from build123d import *

# Parameters (mm, degrees)
F0_W     = 25.3558125973
F0_H     = 19.05
F1_DEPTH = 63.5


with BuildPart() as f1:
    # F0 (on Front) → F1 (new body, symmetric)
    with BuildSketch(Plane.XZ):
        with BuildLine():
            add(Edge.make_bspline(
                [(-41.275, 9.525), (-35.7851044723, 45.3244073821), (12.6259092466, 60.7791905255), (51.7188934867, 61.909732843)],
                knots=[0, 0, 0, 0, 106.3505390395, 106.3505390395, 106.3505390395, 106.3505390395], degree=3))
            Line((-41.275, 9.525), (22.225, 9.525))
            Line((22.225, 9.525), (22.225, 27.4096066543))
            ThreePointArc((22.225, 27.4096066543), (30.6034651981, 50.1040358168), (51.7188934867, 61.909732843))
        make_face()
        Polygon((22.225, 9.525), (-41.275, 9.525), (-41.275, -9.525), (41.275, -9.525), (41.275, 9.525), align=None)
        with BuildLine():
            Line((22.225, 27.4096066543), (22.225, 9.525))
            Line((22.225, 9.525), (41.275, 9.525))
            Line((41.275, 9.525), (41.275, 27.4096066543))
            ThreePointArc((41.275, 27.4096066543), (44.7225989891, 37.2876291848), (53.567954849, 42.8752))
            Line((53.567954849, 42.8752), (60.325, 42.8752))
            Line((60.325, 42.8752), (60.325, 61.9252))
            Line((60.325, 61.9252), (52.2881304538, 61.9252))
            add(Edge.make_bspline(
                [(51.7188934867, 61.909732843), (51.9088611725, 61.9152265783), (52.0986088263, 61.9203820671), (52.2881304538, 61.9252)],
                knots=[106.3505390395, 106.3505390395, 106.3505390395, 106.3505390395, 106.8673367765, 106.8673367765, 106.8673367765, 106.8673367765], degree=3))
            ThreePointArc((51.7188934867, 61.909732843), (30.6034651981, 50.1040358168), (22.225, 27.4096066543))
        make_face()
        with BuildLine():
            ThreePointArc((51.8180734259, 61.9252), (51.7684778995, 61.9175020535), (51.7188934867, 61.909732843))
            add(Edge.make_bspline(
                [(51.7188934867, 61.909732843), (51.9088611725, 61.9152265783), (52.0986088263, 61.9203820671), (52.2881304538, 61.9252)],
                knots=[106.3505390395, 106.3505390395, 106.3505390395, 106.3505390395, 106.8673367765, 106.8673367765, 106.8673367765, 106.8673367765], degree=3))
            Line((52.2881304538, 61.9252), (51.8180734259, 61.9252))
        make_face()
        with BuildLine():
            add(Edge.make_bspline(
                [(52.2881304538, 61.9252), (55.0200364706, 61.994649277), (57.7049776323, 61.993959567), (60.325, 61.9252)],
                knots=[106.8673367765, 106.8673367765, 106.8673367765, 106.8673367765, 114.3168446032, 114.3168446032, 114.3168446032, 114.3168446032], degree=3))
            Line((52.2881304538, 61.9252), (60.325, 61.9252))
        make_face()
        with Locations((73.0029062986, 52.4002)):
            Rectangle(F0_W, F0_H)
        Polygon((60.325, 66.675), (60.325, 61.9252), (85.6808125973, 61.9252), (85.6808125973, 42.8752), (60.325, 42.8752), (60.325, 38.1), (111.125, 38.1), (111.125, 66.675), align=None)
    extrude(amount=F1_DEPTH, both=True)


solid = f1.part
Part model, mm, in its own coordinate system. A direction names the side the tool comes from. Round coordinates to 2 decimals unless told otherwise and drop trailing zeros. Write each loop counter-clockwise with the first axis right and the second up, starting at its lowest first coordinate (ties: lowest second). Pieces come first, ordered by that corner, then holes. Notation, with made-up numbers: M 60.25,62 L 97.25,62 A13 cw 97.25,74 Z; hole C 26,9 d9. An arc over 180 degrees is marked long. Return JSON: item names as keys, results as strings. Group by question number.
(1) Which spindle directions (+Z, -Z, +X, -X, +Y, -Y) get a long thin tool onto all of the face, cutting with end or side? Do faces 5 (the face through (57, -1, 42.875)), 6 (the face through (19, -63.5, 29)), 7 (the face through (85, -1, 38.1)). Say none if no direction does.
(2) Two-plate mould, pull along X, no slides. Class faces 1 (the face through (111.125, -1, 52)), 2 (the face through (60.325, -1, 64)), 3 (the face through (19, 63.5, 29)), 4 (the face through (60.325, -1, 41)): +X half, -X half, draft (parallel to the pull), parting line (faces both ways), or undercut.
(3) Saw through at A-A on x = 93. Write the cut outline in (y, z) (3 decimals), then the cut area to 3 significant figures.
(4) Pin check, flat tips, straight feed: pin 1 Ø1.5 at (x, y) = (11, 30) entering from +Z; pin 2 Ø1.4 at (y, z) = (3.5, 40) entering from -X; pin 3 Ø2.5 at (y, z) = (27, 63.5) entering from -X (3 decimals). Stop position of each tip, or through.
(5) Drill centre lines: probe 1 along Z at (x, y) = (86.5, 42.5) (3 decimals); probe 2 along Z at (x, y) = (56, 32.5); probe 3 along X at (y, z) = (12.5, 40) (3 decimals). Where is each one in solid material? Low to high.
Returned:
{
 "1": {"face 5": "-Z, +Y, -Y", "face 6": "+Z, -Z, +X, -X, -Y", "face 7": "-Z, +X, +Y, -Y"},
 "2": {"face 1": "+X half", "face 2": "-X half", "face 3": "draft", "face 4": "undercut"},
 "3": {"outline": "M -63.5,38.1 L 63.5,38.1 L 63.5,66.675 L -63.5,66.675 Z", "area": "3,630 mm²"},
 "4": {"pin 1": "z = 55.87", "pin 2": "x = -22.74", "pin 3": "x = 60.325"},
 "5": {"probe 1": "38.1 to 66.675", "probe 2": "42.88 to 61.98", "probe 3": "-21.84 to 47.481, 60.325 to 111.125"}
}
